Verification items for the finished model (mm, model axes). Coordinates: 2 decimals unless noted, no trailing zeros. Write each loop counter-clockwise with the first axis right and the second up, starting at its lowest first coordinate (ties: lowest second). Pieces come first, ordered by that corner, then holes. Notation, with made-up numbers: M 76.5,28.25 L 80.5,28.25 A28 ccw 80.5,61.25 Z; hole C -38.5,1 d8. An arc over 180 degrees is marked long. One line per item, written item: value.
```python
from build123d import *

# Parameters (mm, degrees)
BOSS_EXTRUDE2_DEPTH = 2.54
SKETCH7_R           = 1.4986
SKETCH7_W           = 25.4
SKETCH7_H           = 5.08
CUT_EXTRUDE1_DEPTH  = 2.54
CUT_EXTRUDE2_DEPTH  = 47.522645815


with BuildPart() as part:
    # Sketch1 → Boss-Extrude2 (new body)
    with BuildSketch(Plane(origin=(0, 0, 0), x_dir=(1, 0, 0), z_dir=(0, 1, 0))):
        Polygon((3.221868426, 6.029765094), (14.988277627, 17.796174295), (14.988277627, 35.576174295), (-4.295819053, 6.35), (-29.8704, 6.35), (-29.8704, -1.27), (-4.295819053, -1.27), (14.988277627, -30.496174295), (14.988277627, -12.716174295), (3.221868426, -0.949765094), align=None)
    extrude(amount=BOSS_EXTRUDE2_DEPTH)

    # Sketch7 → Cut-Extrude1 (cut)
    with BuildSketch(Plane(origin=(0, 2.54, 0), x_dir=(1, 0, 0), z_dir=(0, 1, 0))):
        with Locations(Location((-27.5844, 2.54, 0), (0, 0, 270))):
            Circle(SKETCH7_R)
        with Locations(Location((12.702277627, 27.956174295, 0), (0, 0, 270))):
            Circle(SKETCH7_R)
        with Locations(Location((12.622030753, 20.33659685, 0), (0, 0, 270))):
            Circle(SKETCH7_R)
        with Locations(Location((12.622030753, -15.25659685, 0), (0, 0, 90))):
            Circle(SKETCH7_R)
        with Locations(Location((12.702277627, -22.876174295, 0), (0, 0, 90))):
            Circle(SKETCH7_R)
        with Locations((-12.5984, 2.54)):
            Rectangle(SKETCH7_W, SKETCH7_H)
    extrude(amount=-CUT_EXTRUDE1_DEPTH, mode=Mode.SUBTRACT)

    # Sketch8 → Cut-Extrude2 (cut, through all)
    with BuildSketch(Plane(origin=(0, 2.54, 0), x_dir=(1, 0, 0), z_dir=(0, 1, 0))):
        Polygon((0.1016, 5.08), (3.221868426, 5.08), (3.221868426, 0), (0, 0), align=None)
    extrude(amount=-CUT_EXTRUDE2_DEPTH, mode=Mode.SUBTRACT)


solid = part.part
```
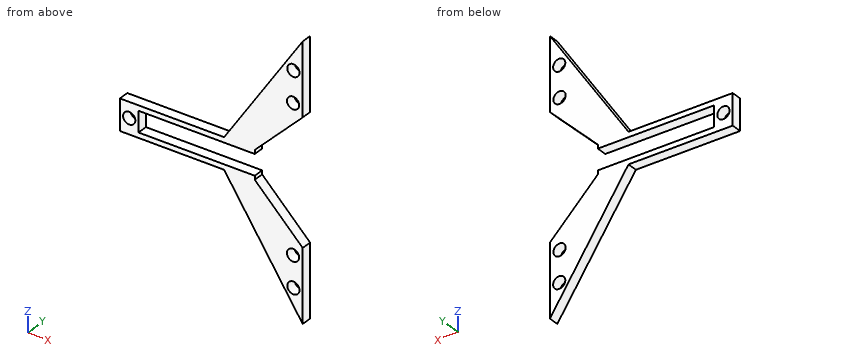
Item 1: Cross-section at B-B, the plane z = -2.54. Enter the section's corners in (x, y).
The answers:
outline: M -29.87,0 L -29.08,0 L -29.08,2.54 L -29.87,2.54 Z; M -26.09,0 L -25.3,0 L -25.3,2.54 L -26.09,2.54 Z
Item 2: Cross-section at D-D, the plane z = -17. Enter the section's corners in (x, y), and give its area (3 significant figures).
The answers:
outline: M 2.73,0 L 14.19,0 L 14.19,2.54 L 2.73,2.54 Z
area: 29.1 mm²
Item 3: Go/stop test with flat-tipped pins: P1, Ø1.5, axis at x = -9.5, z = -2.5, coming from the +Y side; P2, Ø1.5, axis at y = 1.5, z = -23, coming from the -X side; P3, Ø0.8, axis at y = 2, z = -5.5, coming from the +X side; P4, Ø1.3, axis at y = 2, z = -1.5, coming from the +X side. Record where each tip stops, or that it passes through.
The answers:
P1: passes through
P2: stops at x = 6.2
P3: stops at x = 3.22
P4: stops at x = -25.3
Item 4: Scan lines: line 1 (X direction, y = 0.6, z = -2.54); line 2 (Z direction, x = -6, y = 0.4); line 3 (Z direction, x = 3.5, y = 1.45). Record each from-to range of solid material in increasing order.
The answers:
line 1: x = -29.87 to -29.08, -26.09 to -25.3
line 2: z = -6.35 to -5.08, 0 to 1.27
line 3: z = -18.17 to -6.31, 1.23 to 13.09
Item 5: Cross-section at A-A, the plane x = -12. Enter the section's corners in (y, z), and give its area (3 significant figures).
The answers:
outline: M 0,-6.35 L 2.54,-6.35 L 2.54,-5.08 L 0,-5.08 Z; M 0,0 L 2.54,0 L 2.54,1.27 L 0,1.27 Z
area: 6.45 mm²
Item 6: Cross-section at C-C, the plane y = 2.1. Enter the section's corners in (x, z).
The answers:
outline: M -29.87,-6.35 L -4.3,-6.35 L 14.99,-35.58 L 14.99,-17.8 L 3.22,-6.03 L 3.22,-5.08 L -25.3,-5.08 L -25.3,0 L 3.22,0 L 3.22,0.95 L 14.99,12.72 L 14.99,30.5 L -4.3,1.27 L -29.87,1.27 Z; hole C -27.58,-2.54 d3; hole C 12.62,-20.34 d3; hole C 12.62,15.26 d3; hole C 12.7,-27.96 d3; hole C 12.7,22.88 d3
